Work out the finished part from the listing and answer in its coordinate system (mm). A direction names the side the tool comes from. Round coordinates to 2 decimals unless told otherwise and drop trailing zeros. Order: outer loops, then holes, each group sorted by start corner. A loop starts at its lowest first (then second) coordinate and runs counter-clockwise, first axis right, second up. Notation, with made-up numbers: (-31.5, 55) - (19.5, 55) arc R25 ccw to (19.5, 79) - close; hole circle Ø2 at (82, -22.75). An arc over 180 degrees is marked (long way). Use CSV: the item, a comma, the result in double quotes.
from build123d import *

# Parameters (mm, degrees)
SKETCH2_R           = 1.5
BOSS_EXTRUDE1_DEPTH = 5


with BuildPart() as part:
    # Sketch2 → Boss-Extrude1 (new body)
    with BuildSketch(Plane.XY):
        with BuildLine():
            Line((2.786749194, 11.219281361), (1.679332735, 8.620125122))
            ThreePointArc((1.679332735, 8.620125122), (0, 7.492843349), (-1.679332735, 8.620125122))
            Line((-1.679332735, 8.620125122), (-2.166097038, 9.762582836))
            ThreePointArc((-2.166097038, 9.762582836), (-9.883747584, 1.52037288), (-5, -8.660254038))
            Line((-5, -8.660254038), (-5, -33))
            ThreePointArc((-5, -33), (0, -38), (5, -32.999999999))
            Line((5, -32.999999999), (4.999812723, -11.943549515))
            ThreePointArc((4.999812723, -11.943549515), (6.546655646, -9.774570585), (5.060672488, -7.563451711))
            ThreePointArc((5.060672488, -7.563451711), (5.196669714, -5.419737645), (7.282816493, -4.907881363))
            Line((7.282816493, -4.907881363), (10.186929901, -6.110804524))
            ThreePointArc((10.186929901, -6.110804524), (12.473305355, -5.163446511), (11.525947342, -2.877071058))
            Line((11.525947342, -2.877071058), (8.926791103, -1.769654599))
            ThreePointArc((8.926791103, -1.769654599), (7.507129847, -0.157755799), (8.620125937, 1.679333073))
            Line((8.620125937, 1.679333073), (11.524239345, 2.882256233))
            ThreePointArc((11.524239345, 2.882256233), (12.471253953, 5.168928764), (10.18447198, 6.11567907))
            Line((10.18447198, 6.11567907), (7.56352929, 5.060859756))
            ThreePointArc((7.56352929, 5.060859756), (5.419892956, 5.196791944), (4.907881363, 7.282816493))
            Line((4.907881363, 7.282816493), (6.110804524, 10.186929901))
            ThreePointArc((6.110804524, 10.186929901), (5.022287729, 12.549745986), (2.786749194, 11.219281361))
        make_face()
        with Locations((0, -33)):
            Circle(SKETCH2_R, mode=Mode.SUBTRACT)
        Circle(SKETCH2_R, mode=Mode.SUBTRACT)
    extrude(amount=BOSS_EXTRUDE1_DEPTH)


solid = part.part
(1) Find the intervals of material crossed by L1, parallel to Y at x = 0, z = 1.35; L2, parallel to X at y = -14, z = 4.1; L3, parallel to Y at x = 8.25, z = 4, in increasing order. Write a range as from..to.
Findings below:
L1,"y = -38..-34.5, -31.5..-1.5, 1.5..7.49"
L2,"x = -5..5"
L3,"y = -5.31..-1.47, 1.47..5.34"
(2) Each of these flat-tipped pins is pushed along its axis until it touches: pin 1 (3.5 mm diameter, centred on x = 0, y = -33, fed in from +Z); pin 2 (2.5 mm diameter, centred on y = -20, z = 2.5, fed in from -X); pin 3 (2 mm diameter, centred on x = 1, z = 2.5, fed in from +Y); pin 4 (3 mm diameter, centred on x = -4.5, z = 1, fed in from -Y). Where does it stop, or does it pass through?
Findings below:
pin 1,"stops at z = 5"
pin 2,"stops at x = -5"
pin 3,"stops at y = 9.37"
pin 4,"stops at y = -37"
(3) Find section C-C (z = 0.45). Determine the outline of the cut face in (x, y), and give its area (3 significant figures).
Findings below:
outline,"(-5, -33) arc R5 ccw to (5, -33) - (5, -11.94) arc R2.34 ccw to (5.06, -7.56) arc R1.81 cw to (7.28, -4.91) - (10.19, -6.11) arc R1.75 ccw to (11.53, -2.88) - (8.93, -1.77) arc R1.81 cw to (8.62, 1.68) - (11.52, 2.88) arc R1.75 ccw to (10.18, 6.12) - (7.56, 5.06) arc R1.81 cw to (4.91, 7.28) - (6.11, 10.19) arc R1.75 ccw (long way) to (2.79, 11.22) - (1.68, 8.62) arc R1.81 cw to (-1.68, 8.62) - (-2.17, 9.76) arc R10 ccw to (-5, -8.66) - close; hole circle Ø3 at (0, -33); hole circle Ø3 at (0, 0)"
area,"581 mm²"
(4) Find section A-A (y = 0). Determine the outline of the cut face in (x, z).
Findings below:
outline,"(-10, 0) - (-1.5, 0) - (-1.5, 5) - (-10, 5) - close; (1.5, 0) - (7.5, 0) - (7.5, 5) - (1.5, 5) - close"
(5) The mould has two halves that part along Y. Classify faces 4 (the flat face through (10.24, -2.33, 2.46)), 5 (the flat face through (8.9, 5.6, 2.5)), 6 (the flat face through (-1, -12, 0)), 7 (the cylindrical face through (-0.325, -34.464, 2.465)): released by +Y, released by -Y, zero draft, split by the parting line, or undercut.
Findings below:
face 4,"undercut"
face 5,"released by +Y"
face 6,"zero draft"
face 7,"undercut"
(6) Find section B-B (x = 0). Determine the outline of the cut face in (y, z), and give its area (3 significant figures).
Findings below:
outline,"(-38, 0) - (-34.5, 0) - (-34.5, 5) - (-38, 5) - close; (-31.5, 0) - (-1.5, 0) - (-1.5, 5) - (-31.5, 5) - close; (1.5, 0) - (7.49, 0) - (7.49, 5) - (1.5, 5) - close"
area,"197 mm²"
(7) Find section D-D (y = -12.5). Determine the outline of the cut face in (x, z).
Findings below:
outline,"(-5, 0) - (5, 0) - (5, 5) - (-5, 5) - close"
(8) For faces 1 (the cylindrical face through (-9.857, 1.686, 2.465)), 2 (the flat face through (5.5, 8.71, 2.46)), 3 (the flat face through (2.24, 9.94, 2.46)), determine the directions among +Z, -Z, +X, -X, +Y, -Y from which every point of the face is accessible in a straight line to the end or side of a thin tool.
Findings below:
face 1,"+Z, -Z, -X"
face 2,"+Z, -Z, +X"
face 3,"+Z, -Z, +Y"
